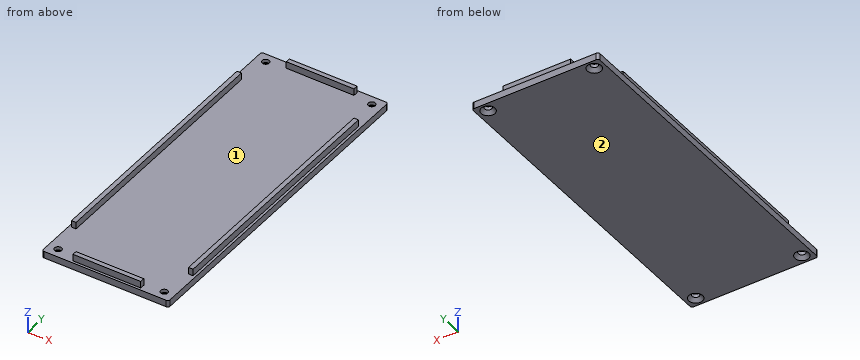
```python
from build123d import *

# Parameters (mm, degrees)
SKETCH_W      = 56
SKETCH_H      = 146
PAD_DEPTH     = 3
SKETCH001_W   = 2
SKETCH001_H   = 110
SKETCH001_W_2 = 30
SKETCH001_H_2 = 2
PAD001_DEPTH  = 3
SKETCH002_R   = 1.55
POCKET_DEPTH  = 3
CHAMFER_SIZE  = 1.5
FILLET_R      = 1


with BuildPart() as part:
    # Sketch → Pad (new body)
    with BuildSketch(Plane.XY):
        Rectangle(SKETCH_W, SKETCH_H)
    extrude(amount=PAD_DEPTH)

    # Sketch001 (on Face6 of Pad) → Pad001 (join)
    with BuildSketch(Plane.XY.offset(3)):
        with Locations((-25.9, 0)):
            Rectangle(SKETCH001_W, SKETCH001_H)
        with Locations((25.9, 0)):
            Rectangle(SKETCH001_W, SKETCH001_H)
        with Locations((0, 70.9)):
            Rectangle(SKETCH001_W_2, SKETCH001_H_2)
        with Locations((0, -70.9)):
            Rectangle(SKETCH001_W_2, SKETCH001_H_2)
    extrude(amount=PAD001_DEPTH)

    # Sketch002 (on Face4 of Pad001) → Pocket (cut)
    with BuildSketch(Plane(origin=(0, 0, 0), x_dir=(1, 0, 0), z_dir=(0, 0, -1))):
        with Locations((-23.5, 69)):
            Circle(SKETCH002_R)
        with Locations((23.5, 69)):
            Circle(SKETCH002_R)
        with Locations((-23.5, -69)):
            Circle(SKETCH002_R)
        with Locations((23.5, -69)):
            Circle(SKETCH002_R)
    extrude(amount=-POCKET_DEPTH, mode=Mode.SUBTRACT)

    # Chamfer
    chamfer_edges = [part.edges().sort_by_distance(p)[0] for p in [
        (-25.05, -69, 0),
        (21.95, -69, 0),
        (-25.05, 69, 0),
        (21.95, 69, 0),
    ]]
    chamfer(chamfer_edges, length=CHAMFER_SIZE)

    # Fillet
    fillet_edges = [part.edges().sort_by_distance(p)[0] for p in [
        (-28, -73, 1.5),
        (28, -73, 1.5),
        (-28, 73, 1.5),
        (28, 73, 1.5),
    ]]
    fillet(fillet_edges, radius=FILLET_R)


solid = part.part
```
Input: part model. Units: mm. Frame: model coordinates. Face numbers are marked on the shaded views. Round coordinates to 2 decimals unless told otherwise and drop trailing zeros. Write each loop counter-clockwise with the first axis right and the second up, starting at its lowest first coordinate (ties: lowest second). Pieces come first, ordered by that corner, then holes. Notation, with made-up numbers: (45, -5.75) - (58, -5.75) arc R19 ccw to (58, 4.25) - close; hole circle Ø4 at (66.5, 65). An arc over 180 degrees is marked (long way). Write item = value, one per line.
(1) Pull-direction query (Y, two-part tool) for the marked faces 1 and 2; classes: +Y half, -Y half, draft (parallel to the pull), parting line (faces both ways), or undercut.
Geometry check:
face_1 = undercut
face_2 = draft
(2) Material intervals for probe 1 along X at (y, z) = (-69, 2.65); probe 2 along Y at (x, z) = (23.5, 1.9); probe 3 along X at (y, z) = (32, 4.05), sorted ascending.
Geometry check:
probe_1 = -28 to -25.05, -21.95 to 21.95, 25.05 to 28
probe_2 = -73 to -70.55, -67.45 to 67.45, 70.55 to 73
probe_3 = -26.9 to -24.9, 24.9 to 26.9
(3) Section query C-C on x = 4.5. Output: boundary loops of the cut face in (y, z), then the cut area to 3 significant figures.
Geometry check:
outline = (-73, 0) - (73, 0) - (73, 3) - (71.9, 3) - (71.9, 6) - (69.9, 6) - (69.9, 3) - (-69.9, 3) - (-69.9, 6) - (-71.9, 6) - (-71.9, 3) - (-73, 3) - close
area = 450 mm^2
(4) Contact query for flat-ended pins moving along their axis: pin 1 Ø3.5 at (x, z) = (2.5, 5) entering from +Y; pin 2 Ø1.6 at (y, z) = (70.5, 4.5) entering from -X; pin 3 Ø5 at (x, y) = (-23.5, 69) entering from -Z. Output: stop coordinate, or through.
Geometry check:
pin_1 = 71.9
pin_2 = -15
pin_3 = 0.55
(5) Section query B-B on y = -41. Output: boundary loops of the cut face in (x, z).
Geometry check:
outline = (-28, 0) - (28, 0) - (28, 3) - (26.9, 3) - (26.9, 6) - (24.9, 6) - (24.9, 3) - (-24.9, 3) - (-24.9, 6) - (-26.9, 6) - (-26.9, 3) - (-28, 3) - close
(6) Section query A-A on x = -23.5. Output: boundary loops of the cut face in (y, z), then the cut area to 3 significant figures.
Geometry check:
outline = (-73, 0) - (-72.05, 0) - (-70.55, 1.5) - (-70.55, 3) - (-73, 3) - close; (-67.45, 1.5) - (-65.95, 0) - (65.95, 0) - (67.45, 1.5) - (67.45, 3) - (-67.45, 3) - close; (70.55, 1.5) - (72.05, 0) - (73, 0) - (73, 3) - (70.55, 3) - close
area = 415 mm^2
